Autodesk Inventor part; units mm, degrees
ref_plane "YZ Plane" through (0, 0, 0) normal (1, 0, 0) x (0, 1, 0)
ref_plane "XZ Plane" through (0, 0, 0) normal (0, 1, 0) x (-1, 0, 0)
ref_plane "XY Plane" through (0, 0, 0) normal (0, 0, 1) x (1, 0, 0)
sketch "Sketch1" plane through (0, 0, 0) normal (0, 0, 1) x (1, 0, 0)
  line L0 (-21, -21) -> (21, -21)
  line L1 (21, -21) -> (21, 21)
  line L2 (21, 21) -> (-21, 21)
  line L3 (-21, 21) -> (-21, -21)
  line L4 (-21, -21) -> (21, 21) construction
  line L5 (21, -21) -> (-21, 21) construction
  line L6 (-18, -18) -> (18, -18)
  line L7 (18, -18) -> (18, 18)
  line L8 (18, 18) -> (-18, 18)
  line L9 (-18, 18) -> (-18, -18)
  line L10 (-18, -18) -> (18, 18) construction
  line L11 (18, -18) -> (-18, 18) construction
  line L12 (18, 18) -> (13.26, 18)
  line L13 (13.26, 18) -> (13.26, 13.26)
  line L14 (13.26, 13.26) -> (18, 13.26)
  line L15 (18, 13.26) -> (18, 18)
  line L16 (18, 18) -> (14.885, 18)
  line L17 (14.885, 18) -> (14.885, 14.885)
  line L18 (14.885, 14.885) -> (18, 14.885)
  line L19 (18, 14.885) -> (18, 18)
  circle A0 centre (14.885, 14.885) radius 1.625
  line L20 (18, 18) -> (11.3, 18)
  line L21 (11.3, 18) -> (11.3, 11.3)
  line L22 (11.3, 11.3) -> (18, 11.3)
  line L23 (18, 11.3) -> (18, 18)
  circle A1 centre (13.26, 13.26) radius 1.96
  point P0 (0, 0)
  dimension "d0" = 42
  dimension "d1" = 42
  dimension "d2" = 36
  dimension "d3" = 36
  dimension "d4" = 4.74
  dimension "d5" = 4.74
  dimension "d6" = 3.115
  dimension "d7" = 6.7
  dimension "d8" = 6.7
extrude "Extrusion1" add sketch "Sketch1" along normal blind 2 contours L3 L2 L1 L0 | L22 A1 L14 L7 | L8 L13 A1 L21 | L14 A1 A0 L18 L7 | L22 L21 A1 | A1 L13 L14 | L8 L17 A0 A1 L13 | L18 A0 L17 L8 L7 | L14 A0 A1 | A1 A0 L13 | A0 A1 L17 L18 | L18 L17 A0 | L14 L13 A0 | A0 A1
mirror "Mirror1" about plane through (0, 0, 0) normal (1, 0, 0) of "Extrusion1"
mirror "Mirror2" about plane through (0, 0, 0) normal (0, 1, 0) of "Extrusion1", "Mirror1"
fillet "Fillet1" radius 2.25 4 edges at (-11.3, 11.3, 1) (11.3, 11.3, 1) (11.3, -11.3, 1) (-11.3, -11.3, 1)
sketch "Sketch2" plane through (0, 0, 2) normal (0, 0, 1) x (1, 0, 0)
  line L0 (21, -21) -> (21, 21)
  line L1 (21, 21) -> (14.885, 21)
  line L2 (14.885, 21) -> (14.885, 14.885)
  line L3 (14.885, 14.885) -> (21, 14.885)
  line L4 (21, 14.885) -> (21, 21)
  circle A0 centre (14.885, 14.885) radius 1.625
  point P0 (0, 0)
  dimension "d12" = 6.115
  dimension "d13" = 6.115
  dimension "d14" = 3.25
extrude "Extrusion2" cut sketch "Sketch2" against normal blind 2 contours A0 L2 L3 | L3 L2 A0
mirror "Mirror3" about plane through (0, 0, 0) normal (0, 1, 0) of "Extrusion2"
mirror "Mirror4" about plane through (0, 0, 0) normal (1, 0, 0) of "Extrusion2", "Mirror3"
sketch "Sketch5" plane through (0, 0, 2) normal (0, 0, 1) x (1, 0, 0)
  line L0 (-18, -18) -> (18, -18)
  line L1 (18, -18) -> (18, 18)
  line L2 (18, 18) -> (-18, 18)
  line L3 (-18, 18) -> (-18, -18)
  line L4 (-18, -18) -> (18, 18) construction
  line L5 (18, -18) -> (-18, 18) construction
  line L6 (-19.3, -19.3) -> (19.3, -19.3)
  line L7 (19.3, -19.3) -> (19.3, 19.3)
  line L8 (19.3, 19.3) -> (-19.3, 19.3)
  line L9 (-19.3, 19.3) -> (-19.3, -19.3)
  line L10 (-19.3, -19.3) -> (19.3, 19.3) construction
  line L11 (19.3, -19.3) -> (-19.3, 19.3) construction
  point P0 (0, 0)
  dimension "d26" = 36
  dimension "d27" = 36
  dimension "d28" = 38.6
  dimension "d29" = 38.6
extrude "Extrusion5" add sketch "Sketch5" along normal blind 3
fillet "Fillet2" radius 2 4 edges at (21, -21, 1) (21, 21, 1) (-21, 21, 1) (-21, -21, 1)
properties part number "camerashield2"
Verification items for the finished model (mm, model axes). A direction names the side the tool comes from. Coordinates: 2 decimals unless noted, no trailing zeros. Write each loop counter-clockwise with the first axis right and the second up, starting at its lowest first coordinate (ties: lowest second). Pieces come first, ordered by that corner, then holes. Notation, with made-up numbers: (21.5, -37) - (75.5, -37) arc R12 cw to (75.5, -23) - close; hole circle Ø1 at (-10.5, 34). An arc over 180 degrees is marked (long way). Answer as a JSON object with one key per item and string values.
(1) Cross-section at A-A on y = -6. Record the cut outline in (x, z), plus the area to 3 significant figures.
Report:
{"outline": "(-21, 0) - (-18, 0) - (-18, 5) - (-19.3, 5) - (-19.3, 2) - (-21, 2) - close; (18, 0) - (21, 0) - (21, 2) - (19.3, 2) - (19.3, 5) - (18, 5) - close", "area": "19.8 mm^2"}
(2) Gauge pin test, flat ends, axial feed: pin 1 Ø0.9 at (y, z) = (-6.5, 3) entering from +X; pin 2 Ø3.5 at (x, y) = (14, -16) entering from +Z; pin 3 Ø2.5 at (y, z) = (-6, 3.5) entering from -X. Record the tip position at first contact, or that the pin passes through.
Report:
{"pin 1": "x = 19.3", "pin 2": "z = 2", "pin 3": "x = -19.3"}
(3) Tool access check on faces 1 (the flat face through (15, -13, 2)), 2 (the flat face through (0, 21, 1)), 3 (the flat face through (-11.3, 16, 1)). Record the directions out of +Z, -Z, +X, -X, +Y, -Y that give a thin tool (end or side, any length) a straight path to the whole face; none if there is none.
Report:
{"face 1": "+Z", "face 2": "+Z, -Z, +X, -X, +Y", "face 3": "+Z, -Z"}
(4) Mould release check, pull along Y, two halves, no side actions. Record for faces 4 (the cylindrical face through (20.43, 20.4, 1.01)), 5 (the flat face through (0, -19.3, 3)), 6 (the cylindrical face through (15.63, 13.44, 1.01)), 7 (the flat face through (-19.3, 0, 3)): pulls with the +Y half, pulls with the -Y half, needs draft (parallel to the pull), parting line crosses it, or undercut.
Report:
{"face 4": "pulls with the +Y half", "face 5": "pulls with the -Y half", "face 6": "undercut", "face 7": "needs draft"}
(5) Cross-section at D-D on x = -15.5. Record the cut outline in (y, z), plus the area to 3 significant figures.
Report:
{"outline": "(-21, 0) - (-16.39, 0) - (-16.39, 2) - (-18, 2) - (-18, 5) - (-19.3, 5) - (-19.3, 2) - (-21, 2) - close; (-13.38, 0) - (-11.3, 0) - (-11.3, 2) - (-13.38, 2) - close; (11.3, 0) - (13.38, 0) - (13.38, 2) - (11.3, 2) - close; (16.39, 0) - (21, 0) - (21, 2) - (19.3, 2) - (19.3, 5) - (18, 5) - (18, 2) - (16.39, 2) - close", "area": "34.6 mm^2"}
(6) Cross-section at C-C on z = 4.2. Record the cut outline in (x, y), plus the area to 3 significant figures.
Report:
{"outline": "(-19.3, -19.3) - (19.3, -19.3) - (19.3, 19.3) - (-19.3, 19.3) - close; hole (-18, -18) - (18, -18) - (18, 18) - (-18, 18) - close", "area": "194 mm^2"}
(7) Thickness scan on line 1 along Y through (x, z) = (3, 2.35); line 2 along Y through (x, z) = (4.5, 0.8). Record the ranges inside material, lowest first.
Report:
{"line 1": "-19.3 to -18, 18 to 19.3", "line 2": "-21 to -18, 18 to 21"}
